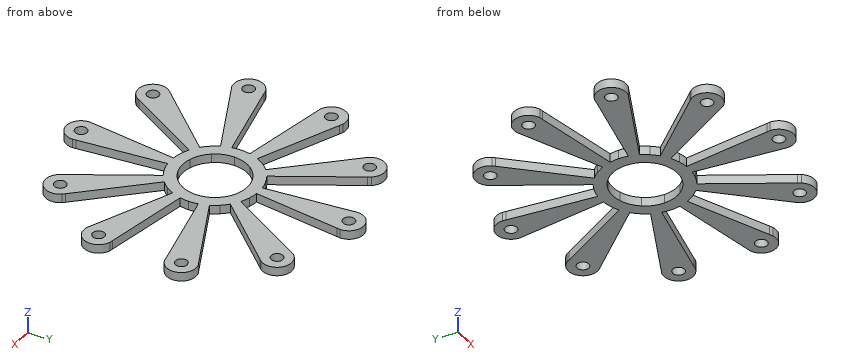
from build123d import *

# Parameters (mm, degrees)
F0_R     = 2
F1_DEPTH = 3


with BuildPart() as f1:
    # F0 (on Top) → F1 (new body)
    with BuildSketch(Plane.XY):
        with BuildLine():
            ThreePointArc((7.422738, 13.034683), (6.060342, 13.721234), (4.635255, 14.265848))
            ThreePointArc((4.635255, 14.265848), (3.162219, 14.662891), (1.656473, 14.908256))
            ThreePointArc((1.656473, 14.908256), (0, 15), (-1.656473, 14.908256))
            ThreePointArc((-1.656473, 14.908256), (-3.162219, 14.662891), (-4.635255, 14.265848))
            ThreePointArc((-4.635255, 14.265848), (-6.060342, 13.721234), (-7.422738, 13.034683))
            ThreePointArc((-7.422738, 13.034683), (-8.816779, 12.135255), (-10.102968, 11.087382))
            ThreePointArc((-10.102968, 11.087382), (-11.17692, 10.003822), (-12.135255, 8.816779))
            ThreePointArc((-12.135255, 8.816779), (-12.968058, 7.538532), (-13.666716, 6.182304))
            ThreePointArc((-13.666716, 6.182304), (-14.265848, 4.635255), (-14.690472, 3.031505))
            ThreePointArc((-14.690472, 3.031505), (-14.922417, 1.523633), (-15, 0))
            ThreePointArc((-15, 0), (-14.922417, -1.523633), (-14.690472, -3.031505))
            ThreePointArc((-14.690472, -3.031505), (-14.265848, -4.635255), (-13.666716, -6.182304))
            ThreePointArc((-13.666716, -6.182304), (-12.968058, -7.538532), (-12.135255, -8.816779))
            ThreePointArc((-12.135255, -8.816779), (-11.17692, -10.003822), (-10.102968, -11.087382))
            ThreePointArc((-10.102968, -11.087382), (-8.816779, -12.135255), (-7.422738, -13.034683))
            ThreePointArc((-7.422738, -13.034683), (-6.060342, -13.721234), (-4.635255, -14.265848))
            ThreePointArc((-4.635255, -14.265848), (-3.162219, -14.662891), (-1.656473, -14.908256))
            ThreePointArc((-1.656473, -14.908256), (0, -15), (1.656473, -14.908256))
            ThreePointArc((1.656473, -14.908256), (3.162219, -14.662891), (4.635255, -14.265848))
            ThreePointArc((4.635255, -14.265848), (6.060342, -13.721234), (7.422738, -13.034683))
            ThreePointArc((7.422738, -13.034683), (8.816779, -12.135255), (10.102968, -11.087382))
            ThreePointArc((10.102968, -11.087382), (11.17692, -10.003822), (12.135255, -8.816779))
            ThreePointArc((12.135255, -8.816779), (12.968058, -7.538532), (13.666716, -6.182304))
            ThreePointArc((13.666716, -6.182304), (14.265848, -4.635255), (14.690472, -3.031505))
            ThreePointArc((14.690472, -3.031505), (14.922417, -1.523633), (15, 0))
            ThreePointArc((15, 0), (14.922417, 1.523633), (14.690472, 3.031505))
            ThreePointArc((14.690472, 3.031505), (14.265848, 4.635255), (13.666716, 6.182304))
            ThreePointArc((13.666716, 6.182304), (12.968058, 7.538532), (12.135255, 8.816779))
            ThreePointArc((12.135255, 8.816779), (11.17692, 10.003822), (10.102968, 11.087382))
            ThreePointArc((10.102968, 11.087382), (8.816779, 12.135255), (7.422738, 13.034683))
        make_face()
        with BuildLine():
            ThreePointArc((-3.399187, 10.461622), (0, 11), (3.399187, 10.461622))
            ThreePointArc((3.399187, 10.461622), (6.465638, 8.899187), (8.899187, 6.465638))
            ThreePointArc((8.899187, 6.465638), (10.461622, 3.399187), (11, 0))
            ThreePointArc((11, 0), (10.461622, -3.399187), (8.899187, -6.465638))
            ThreePointArc((8.899187, -6.465638), (6.465638, -8.899187), (3.399187, -10.461622))
            ThreePointArc((3.399187, -10.461622), (0, -11), (-3.399187, -10.461622))
            ThreePointArc((-3.399187, -10.461622), (-6.465638, -8.899187), (-8.899187, -6.465638))
            ThreePointArc((-8.899187, -6.465638), (-10.461622, -3.399187), (-11, 0))
            ThreePointArc((-11, 0), (-10.461622, 3.399187), (-8.899187, 6.465638))
            ThreePointArc((-8.899187, 6.465638), (-6.465638, 8.899187), (-3.399187, 10.461622))
        make_face(mode=Mode.SUBTRACT)
        with BuildLine():
            ThreePointArc((-1.656473, 14.908256), (0, 15), (1.656473, 14.908256))
            Line((1.656473, 14.908256), (4.878049, 43.902439))
            Line((4.878049, 43.902439), (5, 45))
            ThreePointArc((5, 45), (0, 50), (-5, 45))
            Line((-5, 45), (-4.878049, 43.902439))
            Line((-4.878049, 43.902439), (-1.656473, 14.908256))
        make_face()
        with Locations((0, 45)):
            Circle(F0_R, mode=Mode.SUBTRACT)
        with BuildLine():
            Line((21.858782, 38.385064), (7.422738, 13.034683))
            ThreePointArc((7.422738, 13.034683), (8.816779, 12.135255), (10.102968, 11.087382))
            Line((10.102968, 11.087382), (29.751631, 32.650574))
            Line((29.751631, 32.650574), (30.495421, 33.466838))
            ThreePointArc((30.495421, 33.466838), (29.389263, 40.45085), (22.405251, 39.344691))
            Line((22.405251, 39.344691), (21.858782, 38.385064))
        make_face()
        with Locations((26.450336, 36.405765)):
            Circle(F0_R, mode=Mode.SUBTRACT)
        with BuildLine():
            Line((5, 45), (4.878049, 43.902439))
            ThreePointArc((4.878049, 43.902439), (4.969419, 44.447842), (5, 45))
        make_face()
        with BuildLine():
            ThreePointArc((22.405251, 39.344691), (22.105442, 38.880011), (21.858782, 38.385064))
            Line((21.858782, 38.385064), (22.405251, 39.344691))
        make_face()
        with BuildLine():
            ThreePointArc((-5, 45), (-4.969419, 44.447842), (-4.878049, 43.902439))
            Line((-4.878049, 43.902439), (-5, 45))
        make_face()
        with BuildLine():
            Line((30.495421, 33.466838), (29.751631, 32.650574))
            ThreePointArc((29.751631, 32.650574), (30.14613, 33.038109), (30.495421, 33.466838))
        make_face()
        with BuildLine():
            ThreePointArc((-10.102968, 11.087382), (-8.816779, 12.135255), (-7.422738, 13.034683))
            Line((-7.422738, 13.034683), (-21.858782, 38.385064))
            Line((-21.858782, 38.385064), (-22.405251, 39.344691))
            ThreePointArc((-22.405251, 39.344691), (-29.389263, 40.45085), (-30.495421, 33.466838))
            Line((-30.495421, 33.466838), (-29.751631, 32.650574))
            Line((-29.751631, 32.650574), (-10.102968, 11.087382))
        make_face()
        with Locations((-26.450336, 36.405765)):
            Circle(F0_R, mode=Mode.SUBTRACT)
        with BuildLine():
            Line((40.246301, 18.2059), (13.666716, 6.182304))
            ThreePointArc((13.666716, 6.182304), (14.265848, 4.635255), (14.690472, 3.031505))
            Line((14.690472, 3.031505), (43.261101, 8.9273))
            Line((43.261101, 8.9273), (44.342628, 9.150482))
            ThreePointArc((44.342628, 9.150482), (47.552826, 15.45085), (41.252458, 18.661047))
            Line((41.252458, 18.661047), (40.246301, 18.2059))
        make_face()
        with Locations((42.797543, 13.905765)):
            Circle(F0_R, mode=Mode.SUBTRACT)
        with BuildLine():
            Line((-22.405251, 39.344691), (-21.858782, 38.385064))
            ThreePointArc((-21.858782, 38.385064), (-22.105442, 38.880011), (-22.405251, 39.344691))
        make_face()
        with BuildLine():
            ThreePointArc((41.252458, 18.661047), (40.736775, 18.461337), (40.246301, 18.2059))
            Line((40.246301, 18.2059), (41.252458, 18.661047))
        make_face()
        with BuildLine():
            ThreePointArc((-30.495421, 33.466838), (-30.14613, 33.038109), (-29.751631, 32.650574))
            Line((-29.751631, 32.650574), (-30.495421, 33.466838))
        make_face()
        with BuildLine():
            Line((44.342628, 9.150482), (43.261101, 8.9273))
            ThreePointArc((43.261101, 8.9273), (43.808045, 9.008941), (44.342628, 9.150482))
        make_face()
        with BuildLine():
            ThreePointArc((-14.690472, 3.031505), (-14.265848, 4.635255), (-13.666716, 6.182304))
            Line((-13.666716, 6.182304), (-40.246301, 18.2059))
            Line((-40.246301, 18.2059), (-41.252458, 18.661047))
            ThreePointArc((-41.252458, 18.661047), (-47.552826, 15.45085), (-44.342628, 9.150482))
            Line((-44.342628, 9.150482), (-43.261101, 8.9273))
            Line((-43.261101, 8.9273), (-14.690472, 3.031505))
        make_face()
        with Locations((-42.797543, 13.905765)):
            Circle(F0_R, mode=Mode.SUBTRACT)
        with BuildLine():
            Line((43.261101, -8.9273), (14.690472, -3.031505))
            ThreePointArc((14.690472, -3.031505), (14.265848, -4.635255), (13.666716, -6.182304))
            Line((13.666716, -6.182304), (40.246301, -18.2059))
            Line((40.246301, -18.2059), (41.252458, -18.661047))
            ThreePointArc((41.252458, -18.661047), (47.552826, -15.45085), (44.342628, -9.150482))
            Line((44.342628, -9.150482), (43.261101, -8.9273))
        make_face()
        with Locations((42.797543, -13.905765)):
            Circle(F0_R, mode=Mode.SUBTRACT)
        with BuildLine():
            Line((-41.252458, 18.661047), (-40.246301, 18.2059))
            ThreePointArc((-40.246301, 18.2059), (-40.736775, 18.461337), (-41.252458, 18.661047))
        make_face()
        with BuildLine():
            ThreePointArc((44.342628, -9.150482), (43.808045, -9.008941), (43.261101, -8.9273))
            Line((43.261101, -8.9273), (44.342628, -9.150482))
        make_face()
        with BuildLine():
            ThreePointArc((-44.342628, 9.150482), (-43.808045, 9.008941), (-43.261101, 8.9273))
            Line((-43.261101, 8.9273), (-44.342628, 9.150482))
        make_face()
        with BuildLine():
            Line((41.252458, -18.661047), (40.246301, -18.2059))
            ThreePointArc((40.246301, -18.2059), (40.736775, -18.461337), (41.252458, -18.661047))
        make_face()
        with BuildLine():
            ThreePointArc((-13.666716, -6.182304), (-14.265848, -4.635255), (-14.690472, -3.031505))
            Line((-14.690472, -3.031505), (-43.261101, -8.9273))
            Line((-43.261101, -8.9273), (-44.342628, -9.150482))
            ThreePointArc((-44.342628, -9.150482), (-47.552826, -15.45085), (-41.252458, -18.661047))
            Line((-41.252458, -18.661047), (-40.246301, -18.2059))
            Line((-40.246301, -18.2059), (-13.666716, -6.182304))
        make_face()
        with Locations((-42.797543, -13.905765)):
            Circle(F0_R, mode=Mode.SUBTRACT)
        with BuildLine():
            Line((29.751631, -32.650574), (10.102968, -11.087382))
            ThreePointArc((10.102968, -11.087382), (8.816779, -12.135255), (7.422738, -13.034683))
            Line((7.422738, -13.034683), (21.858782, -38.385064))
            Line((21.858782, -38.385064), (22.405251, -39.344691))
            ThreePointArc((22.405251, -39.344691), (29.389263, -40.45085), (30.495421, -33.466838))
            Line((30.495421, -33.466838), (29.751631, -32.650574))
        make_face()
        with Locations((26.450336, -36.405765)):
            Circle(F0_R, mode=Mode.SUBTRACT)
        with BuildLine():
            Line((-44.342628, -9.150482), (-43.261101, -8.9273))
            ThreePointArc((-43.261101, -8.9273), (-43.808045, -9.008941), (-44.342628, -9.150482))
        make_face()
        with BuildLine():
            ThreePointArc((30.495421, -33.466838), (30.14613, -33.038109), (29.751631, -32.650574))
            Line((29.751631, -32.650574), (30.495421, -33.466838))
        make_face()
        with BuildLine():
            ThreePointArc((-41.252458, -18.661047), (-40.736775, -18.461337), (-40.246301, -18.2059))
            Line((-40.246301, -18.2059), (-41.252458, -18.661047))
        make_face()
        with BuildLine():
            Line((22.405251, -39.344691), (21.858782, -38.385064))
            ThreePointArc((21.858782, -38.385064), (22.105442, -38.880011), (22.405251, -39.344691))
        make_face()
        with BuildLine():
            ThreePointArc((-7.422738, -13.034683), (-8.816779, -12.135255), (-10.102968, -11.087382))
            Line((-10.102968, -11.087382), (-29.751631, -32.650574))
            Line((-29.751631, -32.650574), (-30.495421, -33.466838))
            ThreePointArc((-30.495421, -33.466838), (-29.389263, -40.45085), (-22.405251, -39.344691))
            Line((-22.405251, -39.344691), (-21.858782, -38.385064))
            Line((-21.858782, -38.385064), (-7.422738, -13.034683))
        make_face()
        with Locations((-26.450336, -36.405765)):
            Circle(F0_R, mode=Mode.SUBTRACT)
        with BuildLine():
            Line((4.878049, -43.902439), (1.656473, -14.908256))
            ThreePointArc((1.656473, -14.908256), (0, -15), (-1.656473, -14.908256))
            Line((-1.656473, -14.908256), (-4.878049, -43.902439))
            Line((-4.878049, -43.902439), (-5, -45))
            ThreePointArc((-5, -45), (0, -50), (5, -45))
            Line((5, -45), (4.878049, -43.902439))
        make_face()
        with Locations((0, -45)):
            Circle(F0_R, mode=Mode.SUBTRACT)
        with BuildLine():
            Line((-30.495421, -33.466838), (-29.751631, -32.650574))
            ThreePointArc((-29.751631, -32.650574), (-30.14613, -33.038109), (-30.495421, -33.466838))
        make_face()
        with BuildLine():
            ThreePointArc((5, -45), (4.969419, -44.447842), (4.878049, -43.902439))
            Line((4.878049, -43.902439), (5, -45))
        make_face()
        with BuildLine():
            ThreePointArc((-22.405251, -39.344691), (-22.105442, -38.880011), (-21.858782, -38.385064))
            Line((-21.858782, -38.385064), (-22.405251, -39.344691))
        make_face()
        with BuildLine():
            Line((-5, -45), (-4.878049, -43.902439))
            ThreePointArc((-4.878049, -43.902439), (-4.969419, -44.447842), (-5, -45))
        make_face()
    extrude(amount=F1_DEPTH)


solid = f1.part
For this review, take the finished solid that the model builds, in its own axes (mm). Round coordinates to 2 decimals unless told otherwise and drop trailing zeros. Write each loop counter-clockwise with the first axis right and the second up, starting at its lowest first coordinate (ties: lowest second). Pieces come first, ordered by that corner, then holes. Notation, with made-up numbers: (36.5, 86.5) - (45.5, 86.5) arc R27 ccw to (45.5, 113.5) - close; hole circle Ø4 at (-3.5, 7.5). An arc over 180 degrees is marked (long way). Write item = value, one per line. Start each with the question number.
1. Consider section D-D on x = -20. State the section outline as (y, z) points.
2. Consider section B-B on y = 4.5. State the section outline as (x, z) points.
3. Consider section C-C on y = 27.5. State the section outline as (x, z) points.
4. Consider section A-A on x = 0. State the section outline as (y, z) points, plus the area to 3 significant figures.
5. Wall thickness on L1, parallel to X at y = 40.5, z = 0.1; L2, parallel to Y at x = 13.5, z = 2.3; L3, parallel to X at y = -22.5, z = 1.95: over which ranges is each line inside the solid? List them lowest first.
Evaluation:
q1.outline = (-35.12, 0) - (-21.95, 0) - (-21.95, 3) - (-35.12, 3) - close; (-9.05, 0) - (-4.13, 0) - (-4.13, 3) - (-9.05, 3) - close; (4.13, 0) - (9.05, 0) - (9.05, 3) - (4.13, 3) - close; (21.95, 0) - (35.12, 0) - (35.12, 3) - (21.95, 3) - close
q2.outline = (-21.81, 0) - (-10.04, 0) - (-10.04, 3) - (-21.81, 3) - close; (10.04, 0) - (21.81, 0) - (21.81, 3) - (10.04, 3) - close
q3.outline = (-25.06, 0) - (-15.66, 0) - (-15.66, 3) - (-25.06, 3) - close; (-3.06, 0) - (3.06, 0) - (3.06, 3) - (-3.06, 3) - close; (15.66, 0) - (25.06, 0) - (25.06, 3) - (15.66, 3) - close
q4.outline = (-50, 0) - (-47, 0) - (-47, 3) - (-50, 3) - close; (-43, 0) - (-11, 0) - (-11, 3) - (-43, 3) - close; (11, 0) - (43, 0) - (43, 3) - (11, 3) - close; (47, 0) - (50, 0) - (50, 3) - (47, 3) - close
q4.area = 210 mm2
q5.L1 = -29.32 to -23.58, -4.5 to 4.5, 23.58 to 29.32
q5.L2 = -23.71 to -14.82, -6.54 to 6.54, 14.82 to 23.71
q5.L3 = -20.5 to -12.81, -2.5 to 2.5, 12.81 to 20.5
